Model file for the job. Use its own axes, mm. Face numbers are marked on the shaded views. A direction names the side the tool comes from. Give positions to 0.01 mm unless a question says otherwise; leave off trailing zeros. Loops run counter-clockwise (first coordinate to the right, second up) from the corner with the lowest first, then second, coordinate; pieces in that order, holes last. Notation, with made-up numbers: M -12,41.25 L -3,41.25 A29 cw -3,77.25 Z; hole C 28.5,71 d6. An arc over 180 degrees is marked long. Answer in a Markdown table with one row per item.
```python
from build123d import *

# Parameters (mm, degrees)
BODY1_W                            = 5.9
BODY1_H                            = 4.8
EXTRUDE_1_DEPTH                    = 6
SKETCH_2_W                         = 4.7
SKETCH_2_H                         = 3.6
CUT_EXTRUDE_1_DEPTH                = 4.2
CHAMFER_1_SIZE                     = 0.35
SKETCH_4_W                         = 0.96
SKETCH_4_H                         = 3.91
CUT_EXTRUDE_3_DEPTH                = 0.45
SKETCH_5_W                         = 0.7
SKETCH_5_H                         = 3.45
CUT_EXTRUDE_4_DEPTH                = 0.4
CUT_EXTRUDE_6_REACH                = 11.688
SKETCH_8_W                         = 0.3
SKETCH_8_H                         = 4.05
CUT_EXTRUDE_7_REACH                = 11.688
SKETCH_15_W                        = 4.7
SKETCH_15_H                        = 1.95
CUT_EXTRUDE_9_DEPTH                = 0.65
CHAMFER_7_SIZE                     = 0.65
SKETCH_10_W                        = 0.5
SKETCH_10_H                        = 2.25
EXTRUDE_2_DEPTH                    = 0.3
CHAMFER_2_SIZE                     = 0.25
EXTRUDE_5_DEPTH                    = 0.95
SWEEP_START                        = 1.7
SWEEP_1_DEPTH                      = 0.5
CHAMFER_8_SIZE                     = 0.1
PATTERN_LINEAR_5_COUNT             = 2
PATTERN_LINEAR_5_PITCH             = 2
CHAMFER_8_OF_PATTERN_LINEAR_5_SIZE = 0.1
SKETCH_18_R                        = 0.05
CUT_EXTRUDE_10_DEPTH               = 3.4


# Read off the part's stored shape, not the designer's step: По траектории1
with BuildPart() as part:
    # Body1 → Бобышка-Вытянуть1 (new body)
    with BuildSketch(Plane(origin=(0, 0, 0), x_dir=(1, 0, 0), z_dir=(0, 1, 0))):
        with Locations((2.95, -2.4)):
            Rectangle(BODY1_W, BODY1_H)
    extrude(amount=EXTRUDE_1_DEPTH)

    # Эскиз2 → Вырез-Вытянуть1 (cut)
    with BuildSketch(Plane(origin=(0, 6, 0), x_dir=(1, 0, 0), z_dir=(0, 1, 0))):
        with Locations((2.95, -2.55)):
            Rectangle(SKETCH_2_W, SKETCH_2_H)
    extrude(amount=-CUT_EXTRUDE_1_DEPTH, mode=Mode.SUBTRACT)

    # Фаска1
    chamfer_1_edges = [part.edges().sort_by_distance(p)[0] for p in [
        (5.3, 6, 2.55),
        (2.95, 6, 0.75),
        (0.6, 6, 2.55),
        (2.95, 6, 4.35),
    ]]
    chamfer(chamfer_1_edges, length=CHAMFER_1_SIZE)

    # Эскиз4 → Вырез-Вытянуть3 (cut)
    with BuildSketch(Plane.XY.offset(4.8)):
        with Locations((1.25, 1.955)):
            Rectangle(SKETCH_4_W, SKETCH_4_H)
        with Locations((4.65, 1.955)):
            Rectangle(SKETCH_4_W, SKETCH_4_H)
    extrude(amount=-CUT_EXTRUDE_3_DEPTH, mode=Mode.SUBTRACT)

    # Эскиз5 → Вырез-Вытянуть4 (cut)
    with BuildSketch(Plane(origin=(0, 0, 4.8), x_dir=(1, 0, 0), z_dir=(0, 1, 0))):
        with Locations((1.95, 3.075)):
            Rectangle(SKETCH_5_W, SKETCH_5_H)
    cut_extrude_4 = extrude(amount=CUT_EXTRUDE_4_DEPTH, mode=Mode.SUBTRACT)

    # Эскиз8 → Вырез-Вытянуть6 (cut, up to next)
    with BuildSketch(Plane.XY.offset(4.8), mode=Mode.PRIVATE) as cut_extrude_6_sk1:
        with Locations((2.95, 3.975)):
            Rectangle(SKETCH_8_W, SKETCH_8_H)
    cut_extrude_6_tool1 = extrude(cut_extrude_6_sk1.sketch, amount=-CUT_EXTRUDE_6_REACH, mode=Mode.PRIVATE) & part.part
    add(cut_extrude_6_tool1.solids().sort_by_distance((2.95, 3.975, 4.8))[0], mode=Mode.SUBTRACT)

    # Эскиз9 → Вырез-Вытянуть7 (cut, up to next)
    with BuildSketch(Plane.ZY, mode=Mode.PRIVATE) as cut_extrude_7_sk1:
        with BuildLine():
            Line((2.42, 6), (3.42, 6))
            Line((3.42, 6), (3.42, 4.5))
            ThreePointArc((3.42, 4.5), (2.92, 4), (2.42, 4.5))
            Line((2.42, 4.5), (2.42, 6))
        make_face()
    cut_extrude_7_tool1 = extrude(cut_extrude_7_sk1.sketch, amount=-CUT_EXTRUDE_7_REACH, mode=Mode.PRIVATE) & part.part
    cut_extrude_7 = cut_extrude_7_tool1.solids().sort_by_distance((0, 5.05036, 2.92))[0]
    add(cut_extrude_7, mode=Mode.SUBTRACT)

    # Зеркальное отражение1: Вырез-Вытянуть7 across plane
    add(cut_extrude_7.mirror(Plane(origin=(2.95, 0, 0), x_dir=(0, 0, 1), z_dir=(1, 0, 0))), mode=Mode.SUBTRACT)

    # Эскиз15 → Вырез-Вытянуть9 (cut)
    with BuildSketch(Plane(origin=(0, 1.8, 0), x_dir=(1, 0, 0), z_dir=(0, 1, 0))):
        with Locations((2.95, -1.725)):
            Rectangle(SKETCH_15_W, SKETCH_15_H)
    extrude(amount=-CUT_EXTRUDE_9_DEPTH, mode=Mode.SUBTRACT)

    # Фаска7
    chamfer_7_edges = [part.edges().sort_by_distance(p)[0] for p in [
        (2.95, 1.15, 2.7),
    ]]
    chamfer(chamfer_7_edges, length=CHAMFER_7_SIZE - 0.0001)  # a hair under: the kernel refuses the full size

    # Эскиз10 → Бобышка-Вытянуть2 (add)
    with BuildSketch(Plane.XY.offset(0.75)):
        with Locations((2.95, 2.275)):
            Rectangle(SKETCH_10_W, SKETCH_10_H)
    extrude(amount=EXTRUDE_2_DEPTH)

    # Фаска2
    chamfer_2_edges = [part.edges().sort_by_distance(p)[0] for p in [
        (2.95, 3.4, 1.05),
    ]]
    chamfer(chamfer_2_edges, length=CHAMFER_2_SIZE)

    # Эскиз17 → Бобышка-Вытянуть5 (add)
    with BuildSketch(Plane.ZY):
        Polygon((0, -1.6), (1.95, -1.6), (3.85, 0), (0, 0), align=None)
    extrude_5 = extrude(amount=-EXTRUDE_5_DEPTH)

    # Зеркальное отражение3: Бобышка-Вытянуть5 across plane
    add(extrude_5.mirror(Plane(origin=(2.95, 0, 0), x_dir=(0, 0, 1), z_dir=(1, 0, 0))))

    # По траектории1 outline → По траектории1 (add)
    with BuildSketch(Plane.YZ.offset(SWEEP_START)):
        with BuildLine():
            add(Edge.make_bspline(
                [(-0.5, 2.45), (-0.5, 2.683362296), (-0.405057001, 2.917735205), (-0.152065654, 3.170726552), (-0.050887811, 3.237723146), (0.166472235, 3.327081743), (0.298557942, 3.349954697), (0.4, 3.35)],
                knots=[0.50998091, 0.50998091, 0.50998091, 0.50998091, 0.55448514, 0.55448514, 0.576737255, 0.576737255, 0.59898937, 0.59898937, 0.59898937, 0.59898937], degree=3))
            Line((-0.5, 2.45), (-0.5, -3.4))
            Line((-0.5, -3.4), (0, -3.4))
            Line((0, -3.4), (0, 2.45))
            add(Edge.make_bspline(
                [(0, 2.45), (0, 2.553716576), (0.042196888, 2.657882313), (0.154637487, 2.770322912), (0.199605417, 2.800099176), (0.296209882, 2.839814108), (0.331279974, 2.849979865), (0.4, 2.85)],
                knots=[0.50998091, 0.50998091, 0.50998091, 0.50998091, 0.55448514, 0.55448514, 0.576737255, 0.576737255, 0.59898937, 0.59898937, 0.59898937, 0.59898937], degree=3))
            Line((0.4, 2.85), (0.4, 3.35))
        make_face()
        with BuildLine():
            Line((1.8, 3.35), (1.8, 2.85))
            add(Edge.make_bspline(
                [(1.8, 2.85), (2.1, 2.85), (2.4, 2.85), (3.466666667, 2.85), (4.233333333, 2.85), (5, 2.85)],
                knots=[0.721036083, 0.721036083, 0.721036083, 0.721036083, 0.799494685, 0.799494685, 1, 1, 1, 1], degree=3))
            Line((5, 2.85), (5, 3.35))
            add(Edge.make_bspline(
                [(1.8, 3.35), (2.1, 3.35), (2.4, 3.35), (3.466666667, 3.35), (4.233333333, 3.35), (5, 3.35)],
                knots=[0.721036083, 0.721036083, 0.721036083, 0.721036083, 0.799494685, 0.799494685, 1, 1, 1, 1], degree=3))
        make_face()
    sweep_1 = extrude(amount=SWEEP_1_DEPTH)

    # Фаска8
    chamfer_8_edges = [part.edges().sort_by_distance(p)[0] for p in [
        (1.95, 5, 2.85),
        (2.2, 5, 3.1),
        (1.95, 5, 3.35),
        (1.7, 5, 3.1),
        (1.95, -0.5, -3.4),
        (2.2, -0.25, -3.4),
        (1.95, 0, -3.4),
        (1.7, -0.25, -3.4),
    ]]
    chamfer(chamfer_8_edges, length=CHAMFER_8_SIZE)

    # Линейный массив5: Вырез-Вытянуть4, По траектории1 ×2
    with Locations(*[(i * PATTERN_LINEAR_5_PITCH, 0, 0) for i in range(1, PATTERN_LINEAR_5_COUNT)]):
        add(cut_extrude_4, mode=Mode.SUBTRACT)
        add(sweep_1)

    # Фаска8 of Линейный массив5
    chamfer_8_of_pattern_linear_5_edges = [part.edges().sort_by_distance(p)[0] for p in [
        (3.95, 5, 2.85),
        (4.2, 5, 3.1),
        (3.95, 5, 3.35),
        (3.7, 5, 3.1),
        (3.95, -0.5, -3.4),
        (4.2, -0.25, -3.4),
        (3.95, 0, -3.4),
        (3.7, -0.25, -3.4),
    ]]
    chamfer(chamfer_8_of_pattern_linear_5_edges, length=CHAMFER_8_OF_PATTERN_LINEAR_5_SIZE)

    # Эскиз18 → Вырез-Вытянуть10 (cut)
    with BuildSketch(Plane(origin=(0, 0, 0), x_dir=(-1, 0, 0), z_dir=(0, 0, -1))):
        with Locations(Location((-1.95, -0.25, 0), (0, 0, 90))):
            Circle(SKETCH_18_R)
    extrude(amount=CUT_EXTRUDE_10_DEPTH, mode=Mode.SUBTRACT)


solid = part.part
```
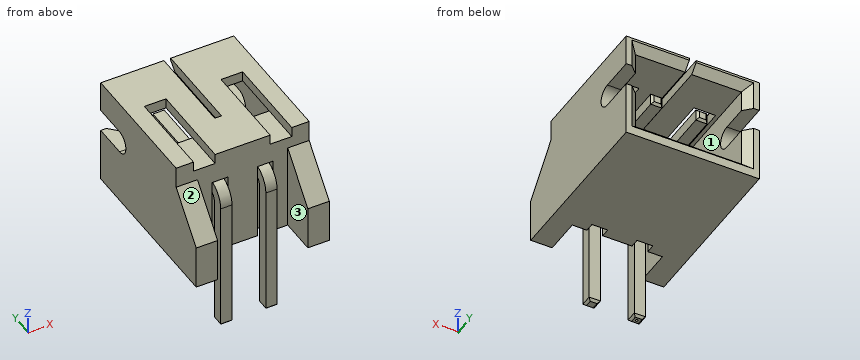
(1) Wall check: L1, parallel to X at y = 0.25, z = 4.5; L2, parallel to X at y = 2.5, z = 1; L3, parallel to Z at x = 3.55, y = 2.5. Give the ranges that are in metal, low to high.
Established:
| item | result |
|---|---|
| L1 | x = 0 to 0.77, 1.73 to 4.17, 5.13 to 5.9 |
| L2 | x = 0 to 0.6, 2.7 to 3.2, 5.3 to 5.9 |
| L3 | z = 0 to 0.75, 4.35 to 4.8 |
(2) Saw through at B-B, the plane x = 5.5. Give the cut face in (y, z).
Established:
| item | result |
|---|---|
| outline | M -1.6,0 L 6,0 L 6,0.4 L 5.85,0.55 L 5.85,2.42 L 4.5,2.42 A0.5 cw 4.5,3.42 L 5.85,3.42 L 5.85,4.55 L 6,4.7 L 6,4.8 L 0,4.8 L 0,3.85 L -1.6,1.95 Z |
(3) Saw through at C-C, the plane y = 2.75. Count the separate pieces of the cut face and the enclosed holes in it, and give its area (3 significant figures).
Established:
| item | result |
|---|---|
| separate pieces | 5 |
| enclosed holes | 0 |
| area | 11.1 mm2 |
(4) Flat gauge pins, fed straight in: P1, Ø0.6, axis at x = 2, z = 2, coming from the -Y side; P2, Ø2, axis at x = 4.5, y = 1, coming from the -Z side. Where does each tip first touch, or does it go through?
Established:
| item | result |
|---|---|
| P1 | stops at y = -0.5 |
| P2 | stops at z = 0 |
(5) Saw through at A-A, the plane z = 4. Give the cut face in (x, y).
Established:
| item | result |
|---|---|
| outline | M 0,0 L 5.9,0 L 5.9,6 L 5.65,6 L 5.3,5.65 L 5.3,1.8 L 0.6,1.8 L 0.6,5.65 L 0.25,6 L 0,6 Z |
(6) Which spindle directions (+Z, -Z, +X, -X, +Y, -Y) get a long thin tool onto all of the face, cutting with end or side? Do the marked faces 1, 2 and 3. Say none if no direction does.
Established:
| item | result |
|---|---|
| face 1 | +Y |
| face 2 | +Z, +X, -X, -Y |
| face 3 | +Z, -Z, -Y |
